Autodesk Inventor part; units mm, degrees
ref_plane "Work Plane1" through (29, 0, 0) normal (0, -1, 0) x (1, 0, 0)
ref_plane "YZ Plane" through (0, 0, 0) normal (1, 0, 0) x (0, 1, 0)
ref_plane "XZ Plane" through (0, 0, 0) normal (0, 1, 0) x (-1, 0, 0)
sketch "Sketch1" plane through (0, 0, 0) normal (0, 0, 1) x (1, 0, 0)
  line L0 (0.2879, 0) -> (9.525, 0)
  line L1 (9.525, 0) -> (9.525, 2.413)
  line L2 (9.525, 2.413) -> (1.5878, 2.413)
  line L3 (1.5878, 2.413) -> (0.0002, 2.413)
  line L4 (0.0002, 2.413) -> (0, 2.413)
  line L5 (0, 2.413) -> (0, 4.5847)
  line L6 (0, 4.5847) -> (-2.5654, 4.5847)
  line L7 (-2.5654, 4.5847) -> (-2.5654, 1.8624)
  line L8 (-2.5654, 1.8624) -> (-0.7874, 1.8624)
  line L9 (-0.7874, 1.8624) -> (0.2879, 0)
  line L10 (-4.9835, 0) -> (11.9431, 0)
  line L11 (0, -0.9169) -> (0, 5.5016)
  line L12 (1.5878, 2.413) -> (0, 2.413) construction
  dimension "d1" = 7.9372
  dimension "d2" = 1.5876
  dimension "d3" = 2.5654
  dimension "d4" = 1.778
  dimension "d5" = 60
  dimension "d6" = 4.826
  dimension "d7" = 4.826
  dimension "d8" = 3.7248
  dimension "d9" = 9.1694
  dimension "d26" = 9.525
revolve "Body" add sketch "Sketch1" angle 360 about axis through (0.2879, 0, 0) along (1, 0, 0) contours L9 L11 L3 L2 L1 L0 | L9 L8 L7 L6 L5 L11
sketch "Sketch2" plane through (-2.5654, 0, 0) normal (-1, 0, 0) x (0, 0, 1)
  circle A0 centre (0, 0) radius 1.8624
  line L0 (0, -6.4186) -> (0, 6.4186)
  line L1 (-6.4186, 0) -> (6.4186, 0)
  line L2 (1.8624, 0) -> (0.9312, -1.6129)
  line L3 (0.9312, -1.6129) -> (-0.9312, -1.6129)
  line L4 (-0.9312, -1.6129) -> (-1.8624, 0)
  line L5 (-1.8624, 0) -> (-0.9312, 1.6129)
  line L6 (-0.9312, 1.6129) -> (0.9312, 1.6129)
  line L7 (0.9312, 1.6129) -> (1.8624, 0)
extrude "Slot" add sketch "Sketch2" against normal up to next contours L7 A0 | A0 L2 | L6 L0 A0 | A0 L0 L3 | L0 L6 A0 | A0 L3 L0 | L4 A0 | A0 L5
fillet "Fillet1" radius 1.778 1 edges at (-2.5654, -4.5847, 0)
thread "Thread"
chamfer "Chamfer1" distance 0.4869 distance2 0.4869 1 edges at (9.525, -2.413, 0) measured on face at (9.525, -0.2686, 0.7084)
ref_plane "Work Plane1" through (29, 0, 0) normal (0, -1, 0) x (1, 0, 0)
fillet "Fillet2" radius 0.1 1 edges at (0.0002, -2.413, 0)
equation "\"d30\" = R"
equation "\"d17\" = RR"
equation "\"d13\" = GEL"
equation "\"d15\" = -0.5 * SPD + 0.5 * GD"
equation "\"d16\" = GUL"
equation "\"d1\" = GEL"
equation "\"d3\" = KOH"
equation "\"d4\" = INTI"
equation "\"d6\" = GD"
equation "\"d7\" = BDM"
equation "\"d8\" = 1.1547 * SW"
equation "\"d9\" = KOD"
equation "\"d26\" = NLG"
equation "\"GD\" = NND"
equation "\"NLG\" = 9.525"
equation "\"GEL\" = 7.93725"
equation "\"KOD\" = 9.1694"
equation "\"KOH\" = 2.5654"
equation "\"INTI\" = 1.778"
equation "\"GAL\" = 1.5875"
equation "\"GUL\" = 0.48692"
equation "\"BDM\" = NND"
equation "\"SW\" = 3.2258"
equation "\"RR\" = 1.778"
equation "\"SPD\" = GD1"
equation "\"R\" = 0.1"
equation "\"KR\" = 4.699"
equation "\"GD1\" = 3.85216"
equation "\"THREADDIA\" = 4.826"
equation "\"FAWI\" = 45deg"
equation "\"KOH1\" = 1.778"
equation "\"NND\" = 4.826"
equation "\"TOA\" = 30deg"
equation "\"E0\" = 1.155 * SW"
properties part number "Unbrako - 10 x 3/8" material "Steel, Mild"
Could you check a few things on this model? Use its own coordinates, in mm. A direction names the side the tool comes from. Coordinates: 2 decimals unless noted, no trailing zeros. Loops run counter-clockwise (first coordinate to the right, second up) from the corner with the lowest first, then second, coordinate; pieces in that order, holes last.
1. For P1, Ø3, axis at x = 4, z = 2.5, coming from the -Y side; P2, Ø0.9, axis at x = -2, z = 0.5, coming from the -Y side; P3, Ø1, axis at y = 1.5, z = -3.5, coming from the -X side, each with a flat end and sliding along its axis, tell me the tip position at first contact or that it passes through.
2. Imagine slicing it at B-B (x = 2). Please give me the cut outline in (y, z).
3. I need wall thicknesses on L1, parallel to Y at x = 2, z = 0; L2, parallel to X at y = 1.25, z = -2.5; L3, parallel to Z at x = 3.25, y = 0.75. Which ranges of each line are inside material? Lowest first, please.
4. For faces 1 (the face through (-2, 1.613, 0)), 2 (the face through (-2.565, -2, 0)), 3 (the face through (0, 3, -1)), which set-ups out of +Z, -Z, +X, -X, +Y, -Y let a thin tool reach every point of the face, with its end or its side?
5. We'd pull the mould along Z, two halves only. Please class faces 4 (the face through (-1.6, -0.8, 1.4)), 5 (the face through (-0.4, -3.64, 2.79)), 6 (the face through (9.525, 0, 0)): released by +Z, released by -Z, zero draft, split by the parting line, or undercut.
6. Imagine slicing it at A-A (x = -1.5). Please give me the cut outline in (y, z).
Computed values:
1. P1: stops at y = -2.2
1. P2: stops at y = -4.39
1. P3: stops at x = -2.49
2. outline: circle Ø4.83 at (0, 0)
3. L1: y = -2.41 to 2.41
3. L2: x = -2.57 to 0
3. L3: z = -2.29 to 2.29
4. face 1: -X
4. face 2: +Z, -Z, -X, +Y, -Y
4. face 3: +X
5. face 4: undercut
5. face 5: split by the parting line
5. face 6: zero draft
6. outline: circle Ø8.87 at (0, 0); hole (-1.61, -0.93) - (0, -1.86) - (1.61, -0.93) - (1.61, 0.93) - (0, 1.86) - (-1.61, 0.93) - close
